Source: CAD feature listing. Evaluate the final solid. Frame: model axes, mm. A direction names the side the tool comes from. Round coordinates to 2 decimals unless told otherwise and drop trailing zeros. Order: outer loops, then holes, each group sorted by start corner. A loop starts at its lowest first (then second) coordinate and runs counter-clockwise, first axis right, second up.
```python
from build123d import *

# Parameters (mm, degrees)
F0_R     = 27.3
F1_DEPTH = 19
F2_R     = 20.7625
F3_DEPTH = 11.5
F4_R     = 18
F5_DEPTH = 7.501
F6_R     = 29.3
F6_R_2   = 27.3
F7_DEPTH = 2.5
F8_SIZE  = 1


with BuildPart() as f1:
    # F0 (on Top) → F1 (new body)
    with BuildSketch(Plane.XY):
        Circle(F0_R)
    extrude(amount=F1_DEPTH)

    # F2 (on face) → F3 (cut)
    with BuildSketch(Plane.XY.offset(19)):
        Circle(F2_R)
    extrude(amount=-F3_DEPTH, mode=Mode.SUBTRACT)

    # F4 (on face) → F5 (cut, through all)
    with BuildSketch(Plane.XY.offset(7.5)):
        Circle(F4_R)
    extrude(amount=-F5_DEPTH, mode=Mode.SUBTRACT)

    # F6 (on face) → F7 (join)
    with BuildSketch(Plane.XY.offset(19)):
        Circle(F6_R)
        Circle(F6_R_2, mode=Mode.SUBTRACT)
    extrude(amount=-F7_DEPTH)

    # F8
    f8_edges = [f1.edges().sort_by_distance(p)[0] for p in [
        (-27.3, 0, 0),
        (-20.7625, 0, 19),
    ]]
    chamfer(f8_edges, length=F8_SIZE)


solid = f1.part
```
1. Section D-D on z = 13.5. Return loops of the section in (x, y) (1 decimal).
2. Pull-direction query (X, two-part tool) for faces 4 (the face through (0, 19, 7.5)), 5 (the face through (0, 22, 19)), 6 (the face through (-21.664, -16.612, 8.642)); classes: released by +X, released by -X, zero draft, split by the parting line, or undercut.
3. Line query: line 1 along Y through (x, z) = (0, 14.5); line 2 along Y through (x, z) = (0, 3.5); line 3 along Z through (x, y) = (17.5, -9). Output: solid intervals per line, ascending.
4. Access query for faces 1 (the face through (26, 9, 16.5)), 2 (the face through (27.947, 8.801, 17.768)), 3 (the face through (19.804, 6.236, 12.824)). Directions: +Z, -Z, +X, -X, +Y, -Y. A direction counts if a zero-diameter tool reaches every point of the face in a straight line with its end or side. Return the directions, or none.
5. Section C-C on z = 6. Return loops of the section in (x, y).
6. Section A-A on x = 0. Return loops of the section in (y, z).
7. First-contact query: pin 1 (3 mm diameter, centred on y = -3, z = 14, fed in from -X); pin 2 (6 mm diameter, centred on y = 8.5, z = 9, fed in from +X); pin 3 (4 mm diameter, centred on x = 3.5, z = 13, fed in from -Y). Flat tips, straight axial feed; report the tip coordinate or a pass-through.
Result:
1. outline: circle Ø54.6 at (0, 0); hole circle Ø41.5 at (0, 0)
2. face 4: undercut
2. face 5: zero draft
2. face 6: split by the parting line
3. line 1: y = -27.3 to -20.76, 20.76 to 27.3
3. line 2: y = -27.3 to -18, 18 to 27.3
3. line 3: z = 0 to 7.5
4. face 1: -Z
4. face 2: +Z, -Z
4. face 3: +Z
5. outline: circle Ø54.6 at (0, 0); hole circle Ø36 at (0, 0)
6. outline: (-29.3, 16.5) - (-27.3, 16.5) - (-27.3, 1) - (-26.3, 0) - (-18, 0) - (-18, 7.5) - (-20.76, 7.5) - (-20.76, 18) - (-21.76, 19) - (-29.3, 19) - close; (18, 0) - (26.3, 0) - (27.3, 1) - (27.3, 16.5) - (29.3, 16.5) - (29.3, 19) - (21.76, 19) - (20.76, 18) - (20.76, 7.5) - (18, 7.5) - close
7. pin 1: stops at x = -27.26
7. pin 2: stops at x = 26.74
7. pin 3: stops at y = -27.26
